Read the model definition and answer for the solid it produces. Units are mm, in the model's axes. A direction names the side the tool comes from. Round coordinates to 2 decimals unless told otherwise and drop trailing zeros. Loops run counter-clockwise (first coordinate to the right, second up) from the corner with the lowest first, then second, coordinate; pieces in that order, holes last. Notation, with made-up numbers: (41, 50.5) - (55, 50.5) arc R14 cw to (55, 65.5) - close; hole circle Ø2 at (86.5, 81). An arc over 180 degrees is marked (long way). Use CSV: the item, a comma, the result in double quotes. Start each with the question number.
1. Consider line 1 along X through (y, z) = (5.5, -0.5); line 2 along Y through (x, z) = (-3, -15.5); line 3 along Y through (x, z) = (6.5, 9.5). Determine where each line is inside the solid, lowest interval first.
2. Find section D-D (z = 7). Give the vertices of the cut face in (x, y), and give its area (3 significant figures).
3. A tool of negligible diameter and unlimited length cuts with its end or side. For faces 4 (the flat face through (2, 10, 0)), 5 (the flat face through (7, 3, -9)), 6 (the cylindrical face through (-11.26, -3.45, 2.17)), from which of +Z, -Z, +X, -X, +Y, -Y can it reach the whole face along a straight path? Write none if from no direction.
4. Find section B-B (x = 4). Give the vertices of the cut face in (y, z), and give its area (3 significant figures).
5. Find section C-C (x = 0). Give the vertices of the cut face in (y, z).
6. Determine the mould class of faces 1 (the cylindrical face through (5.8, 1.38, -0.07)), 2 (the cylindrical face through (9.93, 6.45, 5.38)), 3 (the flat face through (-8, 2.8, 8)) for opening direction Z: +Z half, -Z half, draft (parallel to the pull), parting line (faces both ways), or undercut.
7. Given pin 1 Ø1.5 at (x, z) = (7, -12.5) entering from -Y; pin 2 Ø1 at (y, z) = (-3.5, 5.5) entering from -X; pin 3 Ø6 at (y, z) = (7, 8.5) entering from +X; pin 4 Ø1 at (y, z) = (-1, -11.5) entering from +X, each flat-ended and moving along its own axis, determine where each tip first touches the part or whether it passes through.
8. Find section A-A (z = 0). Give the vertices of the cut face in (x, y), and give its area (3 significant figures).
from build123d import *

# Parameters (mm, degrees)
SKIZZE1_R                        = 18
AUFSATZ_LINEAR_AUSTRAGEN1_DEPTH  = 2.8
SKIZZE2_R                        = 11.5
AUFSATZ_LINEAR_AUSTRAGEN2_DEPTH  = 0.2
SKIZZE3_R                        = 10
AUFSATZ_LINEAR_AUSTRAGEN3_DEPTH  = 7
SKIZZE4_R                        = 10
AUFSATZ_LINEAR_AUSTRAGEN4_DEPTH  = 7
F_3_1_3_1_DURCHMESSER_BOHRUNG1_D = 3.1


with BuildPart() as part:
    # Skizze1 → Aufsatz-Linear austragen1 (new body)
    with BuildSketch(Plane(origin=(0, 0, 0), x_dir=(1, 0, 0), z_dir=(0, 1, 0))):
        with Locations(Location((0, 0, 0), (0, 0, 270))):
            Circle(SKIZZE1_R)
    extrude(amount=AUFSATZ_LINEAR_AUSTRAGEN1_DEPTH)

    # Skizze2 → Aufsatz-Linear austragen2 (add)
    with BuildSketch(Plane(origin=(0, 2.8, 0), x_dir=(1, 0, 0), z_dir=(0, 1, 0))):
        with Locations(Location((1.5, 0, 0), (0, 0, 270))):
            Circle(SKIZZE2_R)
    extrude(amount=AUFSATZ_LINEAR_AUSTRAGEN2_DEPTH)

    # Skizze3 → Aufsatz-Linear austragen3 (add)
    with BuildSketch(Plane(origin=(0, 3, 0), x_dir=(1, 0, 0), z_dir=(0, 1, 0))):
        with Locations(Location((1.5, 0, 0), (0, 0, 270))):
            Circle(SKIZZE3_R)
    extrude(amount=AUFSATZ_LINEAR_AUSTRAGEN3_DEPTH)

    # Skizze4 → Aufsatz-Linear austragen4 (add)
    with BuildSketch(Plane.XZ):
        with Locations(Location((-1.5, 0, 0), (0, 0, 270))):
            Circle(SKIZZE4_R)
    extrude(amount=AUFSATZ_LINEAR_AUSTRAGEN4_DEPTH)

    # Ø3.1 (3.1) Durchmesser Bohrung1 (through all)
    with Locations(Plane(origin=(0, 10, 0), x_dir=(1, 0, 0), z_dir=(0, 1, 0))):
        with Locations((4.25, 0), (-4.25, 0)):
            Hole(F_3_1_3_1_DURCHMESSER_BOHRUNG1_D / 2)


solid = part.part
Filled sheet:
1,line 1,"x = -8.49 to -5.72, -2.78 to 2.78, 5.72 to 11.49"
1,line 2,"y = 0 to 2.8"
1,line 3,"y = 0 to 3"
2,outline,"(-16.58, 0) - (-8.64, 0) - (-8.64, -7) - (5.64, -7) - (5.64, 0) - (16.58, 0) - (16.58, 2.8) - (10.62, 2.8) - (10.62, 3) - (8.64, 3) - (8.64, 10) - (-5.64, 10) - (-5.64, 3) - (-7.62, 3) - (-7.62, 2.8) - (-16.58, 2.8) - close"
2,area,"296 mm²"
3,face 4,"+Z, -Z, +X, -X, +Y"
3,face 5,"+Y"
3,face 6,"-Y"
4,outline,"(-7, -8.35) - (0, -8.35) - (0, -17.55) - (2.8, -17.55) - (2.8, -11.22) - (3, -11.22) - (3, -9.68) - (10, -9.68) - (10, -1.53) - (-7, -1.53) - close; (-7, 1.53) - (10, 1.53) - (10, 9.68) - (3, 9.68) - (3, 11.22) - (2.8, 11.22) - (2.8, 17.55) - (0, 17.55) - (0, 8.35) - (-7, 8.35) - close"
4,area,"303 mm²"
5,outline,"(-7, -9.89) - (0, -9.89) - (0, -18) - (2.8, -18) - (2.8, -11.4) - (3, -11.4) - (3, -9.89) - (10, -9.89) - (10, 9.89) - (3, 9.89) - (3, 11.4) - (2.8, 11.4) - (2.8, 18) - (0, 18) - (0, 9.89) - (-7, 9.89) - close"
6,face 1,"undercut"
6,face 2,"parting line"
6,face 3,"draft"
7,pin 1,"stops at y = 0"
7,pin 2,"stops at x = -10.16"
7,pin 3,"stops at x = 9.85"
7,pin 4,"passes through"
8,outline,"(-18, 0) - (-11.5, 0) - (-11.5, -7) - (-5.8, -7) - (-5.8, 10) - (-8.5, 10) - (-8.5, 3) - (-10, 3) - (-10, 2.8) - (-18, 2.8) - close; (-2.7, -7) - (2.7, -7) - (2.7, 10) - (-2.7, 10) - close; (5.8, -7) - (8.5, -7) - (8.5, 0) - (18, 0) - (18, 2.8) - (13, 2.8) - (13, 3) - (11.5, 3) - (11.5, 10) - (5.8, 10) - close"
8,area,"280 mm²"
